Source: CAD feature listing. Evaluate the final solid. Frame: model axes, mm. Round coordinates to 2 decimals unless told otherwise and drop trailing zeros. Write each loop counter-clockwise with the first axis right and the second up, starting at its lowest first coordinate (ties: lowest second). Pieces come first, ordered by that corner, then holes. Notation, with made-up numbers: M -29,64.25 L 23,64.25 A30 ccw 23,91.25 Z; hole C 36.25,36 d7. An arc over 180 degrees is marked long. Answer in a Markdown table with one row per item.
from build123d import *

# Parameters (mm, degrees)
SKETCH1_W           = 140
SKETCH1_H           = 80
SKETCH1_R           = 2.117
SKETCH1_R_2         = 3.75
SKETCH1_R_3         = 4.5
BOSS_EXTRUDE1_DEPTH = 12
SKETCH2_R           = 3.4
CUT_EXTRUDE1_DEPTH  = 82.510735489
FILLET1_R           = 6


with BuildPart() as part:
    # Sketch1 → Boss-Extrude1 (new body)
    with BuildSketch(Plane.XY):
        Rectangle(SKETCH1_W, SKETCH1_H)
        with Locations((-62.499963671, 32)):
            Circle(SKETCH1_R, mode=Mode.SUBTRACT)
        with Locations((-62.500002371, 20.00021325)):
            Circle(SKETCH1_R_2, mode=Mode.SUBTRACT)
        with Locations((-62.499963671, -32)):
            Circle(SKETCH1_R, mode=Mode.SUBTRACT)
        with Locations((-62.500002371, -19.99978675)):
            Circle(SKETCH1_R_2, mode=Mode.SUBTRACT)
        Circle(SKETCH1_R_3, mode=Mode.SUBTRACT)
        with Locations((62.499963671, 32)):
            Circle(SKETCH1_R, mode=Mode.SUBTRACT)
        with Locations((62.499997629, 20.00021325)):
            Circle(SKETCH1_R_2, mode=Mode.SUBTRACT)
        with Locations((62.499997629, -19.99978675)):
            Circle(SKETCH1_R_2, mode=Mode.SUBTRACT)
        with Locations((62.499963671, -32)):
            Circle(SKETCH1_R, mode=Mode.SUBTRACT)
    extrude(amount=BOSS_EXTRUDE1_DEPTH)

    # Sketch2 → Cut-Extrude1 (cut, through all)
    with BuildSketch(Plane.XY.offset(12)):
        with Locations((42.499997629, 32)):
            Circle(SKETCH2_R)
        with Locations((-42.500002371, 32)):
            Circle(SKETCH2_R)
        with Locations((-42.500002371, 18)):
            Circle(SKETCH2_R)
        with Locations((42.499997629, 18)):
            Circle(SKETCH2_R)
        with Locations((42.499997629, -18)):
            Circle(SKETCH2_R)
        with Locations((42.499997629, -32)):
            Circle(SKETCH2_R)
        with Locations((-42.500002371, -32)):
            Circle(SKETCH2_R)
        with Locations((-42.500002371, -18)):
            Circle(SKETCH2_R)
    extrude(amount=-CUT_EXTRUDE1_DEPTH, mode=Mode.SUBTRACT)

    # Fillet1
    fillet1_edges = [part.edges().sort_by_distance(p)[0] for p in [
        (70, -40, 6),
        (-70, -40, 6),
        (-70, 40, 6),
        (70, 40, 6),
    ]]
    fillet(fillet1_edges, radius=FILLET1_R)

    # Chamfer1
    # the kernel refuses this chamfer: 1 mm, written as the material it takes off along each edge
    with BuildSketch(Plane(origin=(-70, 40.172039171, 12), x_dir=(0.9996219169112968, 0, 0.02749587661058574), z_dir=(0, -1, 0)), Plane(origin=(70, -40.172039171, 12), x_dir=(-0.9996219169112968, 0, 0.02749587661058574), z_dir=(0, 1, 0))) as chamfer1_piece_1:
        with BuildLine():
            Line((1.028673195, 0), (-0.056547155, -1.027117794))
            Line((-0.056547155, -1.027117794), (-0.076539593, -1.026567876))
            ThreePointArc((-0.076539593, -1.026567876), (-0.034129227, -0.51339783), (-0.019992438, 0.000549918))
            Line((-0.019992438, 0.000549918), (0.000549918, 0.019992438))
            ThreePointArc((0.000549918, 0.019992438), (0.514497665, 0.00585565), (1.029223113, 0.019992438))
            Line((1.029223113, 0.019992438), (1.028673195, 0))
        make_face()
    extrude(amount=80.344078342, mode=Mode.SUBTRACT)


solid = part.part
Q1. Section D-D (z = 4). State how many separate pieces and enclosed holes the cut face has, and give its area (3 significant figures).
Solutions:
| item | result |
|---|---|
| separate pieces | 1 |
| enclosed holes | 17 |
| area | 10,600 mm2 |
Q2. Material intervals for probe 1 along X at (y, z) = (-21, 1.5); probe 2 along X at (y, z) = (21.5, 6); probe 3 along X at (y, z) = (32.5, 1), sorted ascending.
Solutions:
| item | result |
|---|---|
| probe 1 | x = -70 to -66.11, -58.89 to -44.1, -40.9 to 40.9, 44.1 to 58.89, 66.11 to 70 |
| probe 2 | x = -70 to -65.94, -59.06 to 59.06, 65.94 to 70 |
| probe 3 | x = -70 to -64.56, -60.44 to -45.86, -39.14 to 39.14, 45.86 to 60.44, 64.56 to 70 |
Q3. Pull-direction query (Y, two-part tool) for faces 1 (the cylindrical face through (60.385, 32.093, 5.916)), 2 (the flat face through (-1, -40, 6)), 3 (the cylindrical face through (-68.289, 38.196, 6.084)); classes: pulls with the +Y half, pulls with the -Y half, needs draft (parallel to the pull), parting line crosses it, or undercut.
Solutions:
| item | result |
|---|---|
| face 1 | undercut |
| face 2 | pulls with the -Y half |
| face 3 | pulls with the +Y half |
Q4. Section B-B (y = 0). Return loops of the section in (x, z).
Solutions:
| item | result |
|---|---|
| outline | M -70,0 L -4.5,0 L -4.5,12 L -69,12 L -70,11 Z; M 4.5,0 L 70,0 L 70,11 L 69,12 L 4.5,12 Z |
Q5. Section A-A (x = 0). Return loops of the section in (y, z), and give its area (3 significant figures).
Solutions:
| item | result |
|---|---|
| outline | M -40,0 L -4.5,0 L -4.5,12 L -40,12 Z; M 4.5,0 L 40,0 L 40,12 L 4.5,12 Z |
| area | 852 mm2 |
Q6. Section C-C (y = -32). Return loops of the section in (x, z), and give its area (3 significant figures).
Solutions:
| item | result |
|---|---|
| outline | M -70,0 L -64.62,0 L -64.62,12 L -69,12 L -70,11 Z; M -60.38,0 L -45.9,0 L -45.9,12 L -60.38,12 Z; M -39.1,0 L 39.1,0 L 39.1,12 L -39.1,12 Z; M 45.9,0 L 60.38,0 L 60.38,12 L 45.9,12 Z; M 64.62,0 L 70,0 L 70,11 L 69,12 L 64.62,12 Z |
| area | 1,410 mm2 |
